Autodesk Inventor part; units mm, degrees
ref_plane "YZ Plane" through (0, 0, 0) normal (1, 0, 0) x (0, 1, 0)
ref_plane "XZ Plane" through (0, 0, 0) normal (0, 1, 0) x (-1, 0, 0)
ref_plane "XY Plane" through (0, 0, 0) normal (0, 0, 1) x (1, 0, 0)
sketch "Skizze1" plane through (0, 0, 0) normal (0, 0, 1) x (1, 0, 0)
  circle A0 centre (0, 0) radius 20
  line L0 (-5.1764, 19.3185) -> (57.5, 36.1126)
  line L1 (-5.1764, -19.3185) -> (57.5, -36.1126)
  circle A1 centre (115, 0) radius 20
  line L2 (57.5, 36.1126) -> (120.1764, 19.3185)
  line L3 (57.5, -36.1126) -> (120.1764, -19.3185)
  circle A2 centre (115, 0) radius 12.5
  circle A3 centre (0, 0) radius 12.5
  dimension "d4" = 40
  dimension "d5" = 25
  dimension "d6" = 25
  dimension "d7" = 115
  dimension "d8" = 57.5
  dimension "d9" = 30
  dimension "d10" = 30
extrude "Extrusion1" add sketch "Skizze1" along normal blind 10
sketch "Skizze2" plane through (0, 0, 10) normal (0, 0, 1) x (1, 0, 0)
  circle A0 centre (57.5, 0) radius 20
  point P0 (0, 0)
  point P1 (57.5, 36.1126)
  dimension "d13" = 40
extrude "Extrusion2" add sketch "Skizze2" along normal blind 60
sketch "Skizze3" plane through (57.5, 0, 70) normal (0, 0, 1) x (1, 0, 0)
  circle A0 centre (0, 0) radius 20
  line L0 (0, 0) -> (0, 5.5377) construction
  circle A1 centre (0, 0) radius 12.5
  point P0 (-57.5, 0)
  dimension "d17" = 25
extrude "Extrusion3" cut sketch "Skizze3" against normal up to surface (70 mm away) contours A1
sketch "Skizze4" plane through (57.5, 0, 70) normal (0, 0, 1) x (1, 0, 0)
  circle A0 centre (0, 0) radius 12.5
  circle A1 centre (0, 0) radius 20
  line L0 (-3, 19.7737) -> (-3, 12.1347)
  line L1 (3, 19.7737) -> (3, 12.1347)
  line L2 (0, 0) -> (0, 16.2882) construction
  circle A2 centre (0, 0) radius 20
  point P0 (-57.5, 0)
  point P1 (3, 19.7737)
  dimension "d20" = 6
extrude "Extrusion4" cut sketch "Skizze4" against normal blind 5 contours A0 L0 A1 L1 picked at (-2.3362, 14.7892)
pattern_circular "Runde Anordnung1" count 4 over 360 about axis through (57.5, 0, 10) along (0, 0, 1) of "Extrusion4"
fillet "Rundung1" radius 35 2 edges at (57.5, 36.1126, 5) (57.5, -36.1126, 5)
equation "\"d6\" = d5"
properties part number "lager_" material "Stahl, galvanisiert"
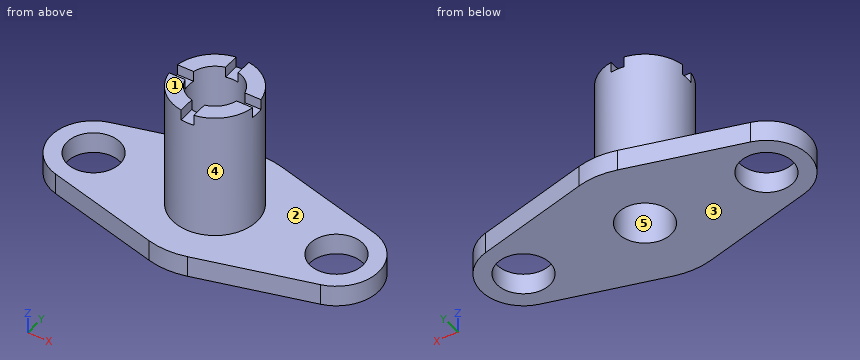
Geometry: final body of the model. Coordinates: model frame, mm. Face numbers are marked on the shaded views. A direction names the side the tool comes from. Give positions to 0.01 mm unless a question says otherwise; leave off trailing zeros. Order: outer loops, then holes, each group sorted by start corner. A loop starts at its lowest first (then second) coordinate and runs counter-clockwise, first axis right, second up. Notation, with made-up numbers: (2.5, 84) -> (9.5, 84) arc R17 cw to (9.5, 101) -> close; hole circle Ø11 at (30.25, 36). An arc over 180 degrees is marked (long way). Answer as a JSON object with one key per item and string values.
Q1. Section D-D (x = 115). Output: boundary loops of the cut face in (y, z), plus the area to 3 significant figures.
Entries:
{"outline": "(-20.71, 0) -> (-12.5, 0) -> (-12.5, 10) -> (-20.71, 10) -> close; (12.5, 0) -> (20.71, 0) -> (20.71, 10) -> (12.5, 10) -> close", "area": "164 mm^2"}
Q2. Draft query along X for the marked faces 3, 4 and 5. Return one class per face: released by +X, released by -X, zero draft, split by the parting line, or undercut.
Entries:
{"face 3": "zero draft", "face 4": "split by the parting line", "face 5": "undercut"}
Q3. Section B-B (y = 0). Output: boundary loops of the cut face in (x, z), plus the area to 4 significant figures.
Entries:
{"outline": "(-20, 0) -> (-12.5, 0) -> (-12.5, 10) -> (-20, 10) -> close; (12.5, 0) -> (45, 0) -> (45, 65) -> (37.5, 65) -> (37.5, 10) -> (12.5, 10) -> close; (70, 0) -> (102.5, 0) -> (102.5, 10) -> (77.5, 10) -> (77.5, 65) -> (70, 65) -> close; (127.5, 0) -> (135, 0) -> (135, 10) -> (127.5, 10) -> close", "area": "1,625 mm^2"}
Q4. Section A-A (x = 57.5). Output: boundary loops of the cut face in (y, z).
Entries:
{"outline": "(-34.88, 0) -> (-12.5, 0) -> (-12.5, 65) -> (-20, 65) -> (-20, 10) -> (-34.88, 10) -> close; (12.5, 0) -> (34.88, 0) -> (34.88, 10) -> (20, 10) -> (20, 65) -> (12.5, 65) -> close"}
Q5. First-contact query: pin 1 (12 mm diameter, centred on y = -14, z = 9, fed in from -X); pin 2 (2 mm diameter, centred on y = 13, z = 47, fed in from +X); pin 3 (5.5 mm diameter, centred on x = 40, z = 66.5, fed in from +Y). Flat tips, straight axial feed; report the tip coordinate or a pass-through.
Entries:
{"pin 1": "stops at x = -18.33", "pin 2": "stops at x = 73.5", "pin 3": "stops at y = 13.51"}
Q6. Access query for the marked faces 1 and 2. Directions: +Z, -Z, +X, -X, +Y, -Y. A direction counts if a zero-diameter tool reaches every point of the face in a straight line with its end or side. Return the directions, or none.
Entries:
{"face 1": "+Z, +X, -X, +Y, -Y", "face 2": "+Z"}
Q7. Material intervals for probe 1 along Y at (x, z) = (57.5, 46); probe 2 along X at (y, z) = (0, 16); probe 3 along Y at (x, z) = (59, 41.5), sorted ascending.
Entries:
{"probe 1": "y = -20 to -12.5, 12.5 to 20", "probe 2": "x = 37.5 to 45, 70 to 77.5", "probe 3": "y = -19.94 to -12.41, 12.41 to 19.94"}
Q8. Section C-C (z = 18). Output: boundary loops of the cut face in (x, y).
Entries:
{"outline": "circle Ø40 at (57.5, 0); hole circle Ø25 at (57.5, 0)"}
